Autodesk Inventor part; units mm, degrees
ref_plane "YZ Plane" through (0, 0, 0) normal (1, 0, 0) x (0, 1, 0)
ref_plane "XZ Plane" through (0, 0, 0) normal (0, 1, 0) x (-1, 0, 0)
ref_plane "XY Plane" through (0, 0, 0) normal (0, 0, 1) x (1, 0, 0)
sketch "Sketch1" plane through (0, 0, 0) normal (0, 0, 1) x (1, 0, 0)
  line L0 (0, 1489.5) -> (-179.3598, 1489.5)
  line L1 (-179.3598, 1489.5) -> (-179.3598, 0)
  line L2 (-179.3598, 0) -> (0, 0)
  line L3 (0, 0) -> (0, 1489.5)
  line L4 (-179.3598, 100) -> (-66, 100)
  line L5 (-66, 100) -> (-66, 105)
  line L6 (-66, 105) -> (-179.3598, 105)
  line L7 (-179.3598, 105) -> (-179.3598, 100)
  line L8 (-179.3598, 596.6667) -> (-66, 596.6667)
  line L9 (-66, 596.6667) -> (-66, 601.6667)
  line L10 (-66, 601.6667) -> (-179.3598, 601.6667)
  line L11 (-179.3598, 601.6667) -> (-179.3598, 596.6667)
  line L12 (-179.3598, 1093.3333) -> (-66, 1093.3333)
  line L13 (-66, 1093.3333) -> (-66, 1098.3333)
  line L14 (-66, 1098.3333) -> (-179.3598, 1098.3333)
  line L15 (-179.3598, 1098.3333) -> (-179.3598, 1093.3333)
  circle A0 centre (-179.3598, 1335) radius 30
  point P0 (-179.3598, 1093.3333)
  point P1 (-179.3598, 596.6667)
  point P2 (-179.3598, 1365)
  point P3 (-179.3598, 1305)
  dimension "d0" = 1489.5
  dimension "d1" = 179.3598
  dimension "d2" = 5
  dimension "d4" = 100
  dimension "d7" = 496.6667
  dimension "d23" = 66
  dimension "d29" = 60
  dimension "d30" = 1335
extrude "Plate1" add sketch "Sketch1" along normal blind 4 contours L3 L2 L1 L4 L5 L6 L8 L9 L10 L12 L13 L14 A0 L0
chamfer "Corner Chamfer1" distance 3 angle 45 6 edges at (-179.3598, 100, 2) (-179.3598, 105, 2) (-179.3598, 596.6667, 2) (-179.3598, 601.6667, 2) (-179.3598, 1098.3333, 2) (-179.3598, 1093.3333, 2)
equation "\"d0\" = Стрингер_длина"
equation "\"d1\" = стрингер_глубина_2"
equation "\"d2\" = паз_под_стрингер_толщина"
equation "\"d7\" = Шаг_шпангоутов"
equation "\"d23\" = паз_под_стрингер_глубина - Thickness"
equation "\"d29\" = 2 * радиус_выреза_под_сварку"
equation "\"d12\" = Thickness"
equation "\"BendRadius\" = Thickness"
equation "\"BendReliefWidth\" = Thickness"
equation "\"BendReliefDepth\" = 0.5 * Thickness"
equation "\"CornerReliefSize\" = 4 * Thickness"
equation "\"MinimumRemnant\" = 2 * Thickness"
equation "\"TransitionRadius\" = BendRadius"
equation "\"JacobiRadiusSize\" = BendRadius"
equation "\"GapSize\" = Thickness"
properties part number "GBK 3114 stringer 2" material "Steel"
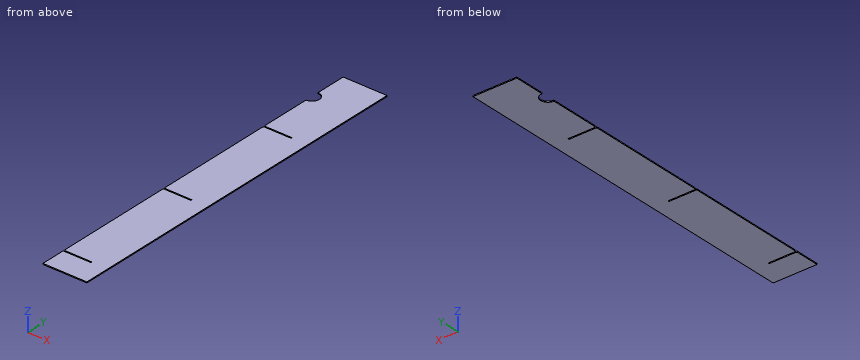
Here's how the part is built. I have some questions about the finished solid (model axes, mm). Coordinates: 2 decimals unless noted, no trailing zeros. Order: outer loops, then holes, each group sorted by start corner. A loop starts at its lowest first (then second) coordinate and runs counter-clockwise, first axis right, second up. Notation, with made-up numbers: (52, 50.5) -> (64, 50.5) arc R17 ccw to (64, 62.5) -> close; hole circle Ø11 at (-29.5, -12). An arc over 180 degrees is marked (long way). Answer in a Markdown table with one row per item.
(1) Will these pins go through, and if not, where does the flat tip stop? pin 1 Ø8 at (x, y) = (-78, 1168.5) entering from -Z; pin 2 Ø1.2 at (y, z) = (1095, 2.5) entering from -X.
Answer key:
| item | result |
|---|---|
| pin 1 | z = 0 |
| pin 2 | x = -66 |
(2) Please list where these lines run through material, in increasing order: probe 1 along Y at (x, z) = (-116.5, 1.9); probe 2 along Y at (x, z) = (-160, 1.65).
Answer key:
| item | result |
|---|---|
| probe 1 | 0 to 100, 105 to 596.67, 601.67 to 1093.33, 1098.33 to 1489.5 |
| probe 2 | 0 to 100, 105 to 596.67, 601.67 to 1093.33, 1098.33 to 1312.08, 1357.92 to 1489.5 |
(3) I want a section at A-A on y = 1335. List the corners of the cut face in (x, z) for me.
Answer key:
| item | result |
|---|---|
| outline | (-149.36, 0) -> (0, 0) -> (0, 4) -> (-149.36, 4) -> close |
